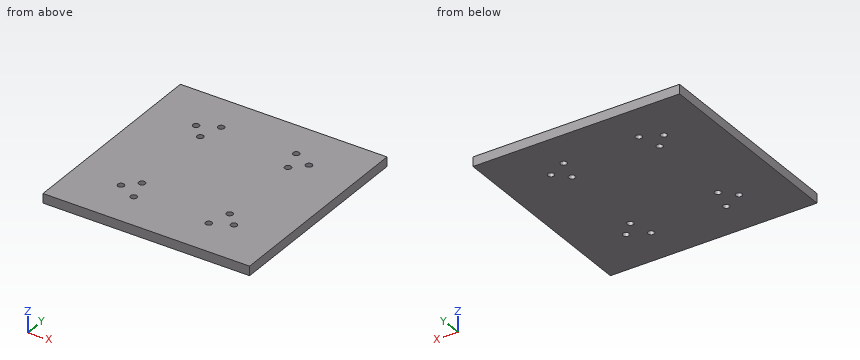
from build123d import *

# Parameters (mm, degrees)
SKIZZE1_W                       = 220
SKIZZE1_H                       = 220
AUFSATZ_LINEAR_AUSTRAGEN1_DEPTH = 10
SKIZZE2_R                       = 3.4
SCHNITT_LINEAR_AUSTRAGEN1_DEPTH = 156.884572681
SKIZZE3_R                       = 3.4
SCHNITT_LINEAR_AUSTRAGEN2_DEPTH = 156.884572681


with BuildPart() as part:
    # Skizze1 → Aufsatz-Linear austragen1 (new body)
    with BuildSketch(Plane.XY):
        Rectangle(SKIZZE1_W, SKIZZE1_H)
    extrude(amount=AUFSATZ_LINEAR_AUSTRAGEN1_DEPTH)

    # Skizze2 → Schnitt-Linear austragen1 (cut, through all)
    with BuildSketch(Plane.XY.offset(10)):
        with Locations((46.669047558, 46.669047558)):
            Circle(SKIZZE2_R)
        with Locations((46.669047558, -46.669047558)):
            Circle(SKIZZE2_R)
        with Locations((-46.669047558, -46.669047558)):
            Circle(SKIZZE2_R)
        with Locations((-46.669047558, 46.669047558)):
            Circle(SKIZZE2_R)
        with Locations((60.104076401, 60.104076401)):
            Circle(SKIZZE2_R)
        with Locations((60.104076401, -60.104076401)):
            Circle(SKIZZE2_R)
        with Locations((-60.104076401, -60.104076401)):
            Circle(SKIZZE2_R)
        with Locations((-60.104076401, 60.104076401)):
            Circle(SKIZZE2_R)
    extrude(amount=-SCHNITT_LINEAR_AUSTRAGEN1_DEPTH, mode=Mode.SUBTRACT)

    # Skizze3 → Schnitt-Linear austragen2 (cut, through all)
    with BuildSketch(Plane.XY.offset(10)):
        with Locations((40, -70)):
            Circle(SKIZZE3_R)
        with Locations(Location((-40, -70, 0), (0, 0, 180))):
            Circle(SKIZZE3_R)
        with Locations(Location((40, 70, 0), (0, 0, 180))):
            Circle(SKIZZE3_R)
        with Locations((-40, 70)):
            Circle(SKIZZE3_R)
    extrude(amount=-SCHNITT_LINEAR_AUSTRAGEN2_DEPTH, mode=Mode.SUBTRACT)


solid = part.part
CAD build for the part. Positions are in the model's coordinates, mm. Give positions to 0.01 mm unless a question says otherwise; leave off trailing zeros. Write each loop counter-clockwise with the first axis right and the second up, starting at its lowest first coordinate (ties: lowest second). Pieces come first, ordered by that corner, then holes. Notation, with made-up numbers: (-6.5, 86) - (16.5, 86) arc R37 ccw to (16.5, 122) - close; hole circle Ø2 at (21, 69). An arc over 180 degrees is marked (long way). Answer as CSV lines item,"result".
Q1. Band-saw the part on B-B (y = -70). Give the cut face in (x, z).
Result set:
outline,"(-110, 0) - (-43.4, 0) - (-43.4, 10) - (-110, 10) - close; (-36.6, 0) - (36.6, 0) - (36.6, 10) - (-36.6, 10) - close; (43.4, 0) - (110, 0) - (110, 10) - (43.4, 10) - close"
Q2. Drill centre lines: line 1 (Y direction, x = 59.5, z = 2.75); line 2 (Y direction, x = 40, z = 8.25); line 3 (X direction, y = 72, z = 4.75). Where is each one in solid material? Low to high. Write a range as from..to.
Result set:
line 1,"-110..-63.45, -56.76..56.76, 63.45..110"
line 2,"-110..-73.4, -66.6..66.6, 73.4..110"
line 3,"-110..-42.75, -37.25..37.25, 42.75..110"
Q3. Flat gauge pin, fed straight in: pin 1 Ø9 at (x, y) = (46.67, 46.67) entering from -Z. Where does the tip first touch, or does it go through?
Result set:
pin 1,"z = 0"
Q4. Band-saw the part on A-A (x = -40). Give the cut face in (y, z), and give its area (3 significant figures).
Result set:
outline,"(-110, 0) - (-73.4, 0) - (-73.4, 10) - (-110, 10) - close; (-66.6, 0) - (66.6, 0) - (66.6, 10) - (-66.6, 10) - close; (73.4, 0) - (110, 0) - (110, 10) - (73.4, 10) - close"
area,"2,060 mm²"
